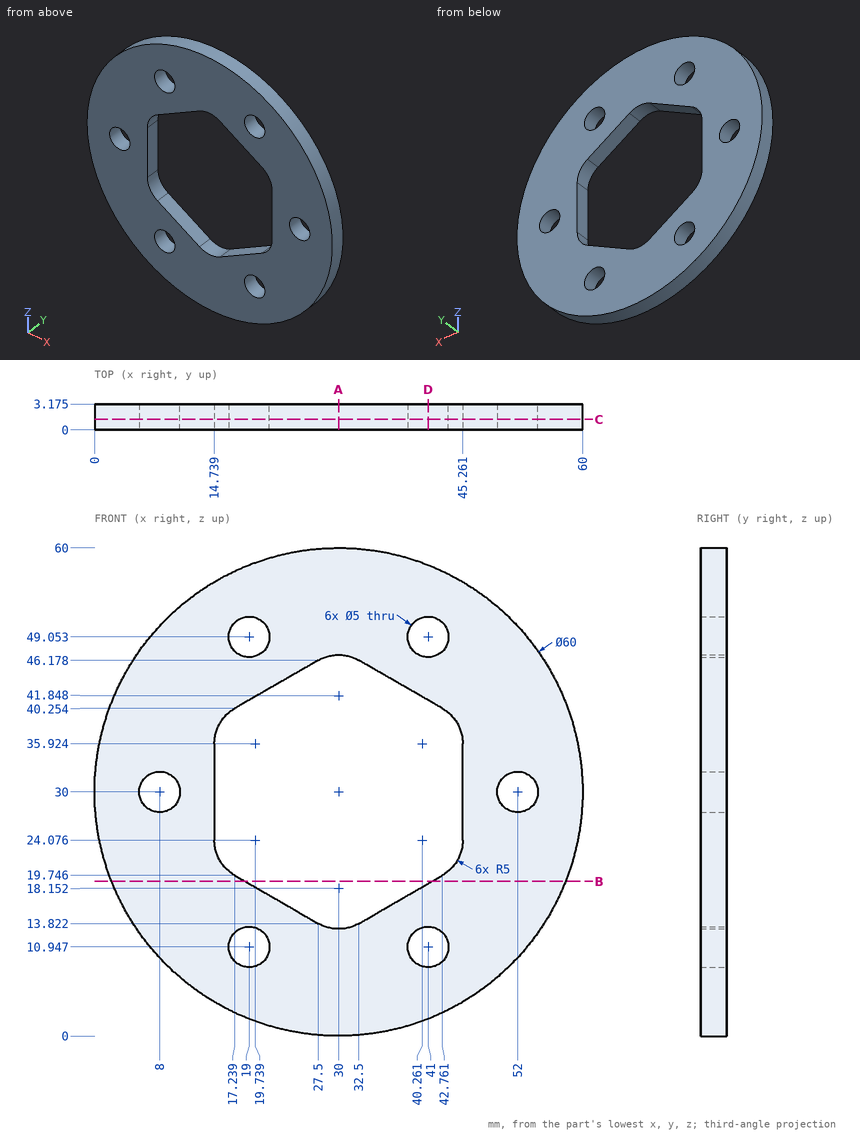
Job drawing, mm, ordinate dimensions from the low corner. One solid piece. Coordinates: 2 decimals unless noted, no trailing zeros. Order: outer loops, then holes, each group sorted by start corner. A loop starts at its lowest first (then second) coordinate and runs counter-clockwise, first axis right, second up. Notation, with made-up numbers: (44.25, 5.5) -> (85.25, 5.5) arc R13 ccw to (85.25, 19.5) -> close; hole circle Ø5 at (63.5, -17). An arc over 180 degrees is marked (long way). Answer in a Markdown table with one row per item. Add a question column.
Q1. Band-saw the part on C-C, the plane y = 1.3. List the corners of the cut face in (x, z) (1 decimal), then the cut area to 3 significant figures.
Q2. Band-saw the part on B-B, the plane z = 19. List the corners of the cut face in (x, y) (1 decimal), then the cut area to 3 significant figures.
Q3. Band-saw the part on A-A, the plane x = 30. List the corners of the cut face in (y, z) (1 decimal).
Q4. Band-saw the part on D-D, the plane x = 41. List the corners of the cut face in (y, z) (1 decimal).
Q5. Drop flat-ended pins along their axis: pin 1 (1 mm diameter, centred on y = 2, z = 31, fed in from -X); pin 2 (1 mm diameter, centred on x = 9.5, y = 3, fed in from +Z); pin 3 (4 mm diameter, centred on x = 19, z = 49.05, fed in from -Y) (3 decimals); pin 4 (1 mm diameter, centred on y = 2, z = 49.5, fed in from -X) (1 decimal). Give the stop position or say it passes through.
Q6. Wall check: line 1 along Z through (x, y) = (19, 0.95); line 2 along X through (y, z) = (1.75, 11) (1 decimal); line 3 along X through (y, z) = (0.9, 28.5). Give the ranges that are in metal, low to high. Write a range as [from, to].
Answers follow:
| question | item | result |
|---|---|---|
| 1 | outline | circle Ø60 at (30, 30); hole circle Ø5 at (8, 30); hole (14.7, 24.1) arc R5 ccw to (17.2, 19.7) -> (27.5, 13.8) arc R5 ccw to (32.5, 13.8) -> (42.8, 19.7) arc R5 ccw to (45.3, 24.1) -> (45.3, 35.9) arc R5 ccw to (42.8, 40.3) -> (32.5, 46.2) arc R5 ccw to (27.5, 46.2) -> (17.2, 40.3) arc R5 ccw to (14.7, 35.9) -> close; hole circle Ø5 at (19, 10.9); hole circle Ø5 at (19, 49.1); hole circle Ø5 at (41, 10.9); hole circle Ø5 at (41, 49.1); hole circle Ø5 at (52, 30) |
| 1 | area | 1,910 mm^2 |
| 2 | outline | (2.1, 0) -> (18.5, 0) -> (18.5, 3.2) -> (2.1, 3.2) -> close; (41.5, 0) -> (57.9, 0) -> (57.9, 3.2) -> (41.5, 3.2) -> close |
| 2 | area | 104 mm^2 |
| 3 | outline | (0, 0) -> (3.2, 0) -> (3.2, 13.2) -> (0, 13.2) -> close; (0, 46.8) -> (3.2, 46.8) -> (3.2, 60) -> (0, 60) -> close |
| 4 | outline | (0, 2.1) -> (3.2, 2.1) -> (3.2, 8.4) -> (0, 8.4) -> close; (0, 13.4) -> (3.2, 13.4) -> (3.2, 18.7) -> (0, 18.7) -> close; (0, 41.3) -> (3.2, 41.3) -> (3.2, 46.6) -> (0, 46.6) -> close; (0, 51.6) -> (3.2, 51.6) -> (3.2, 57.9) -> (0, 57.9) -> close |
| 5 | pin 1 | x = 0 |
| 5 | pin 2 | z = 52.36 |
| 5 | pin 3 | through |
| 5 | pin 4 | x = 6.8 |
| 6 | line 1 | [2.09, 8.45], [13.45, 18.73], [41.27, 46.55], [51.55, 57.91] |
| 6 | line 2 | [6.8, 16.5], [21.5, 38.5], [43.5, 53.2] |
| 6 | line 3 | [0.04, 6], [10, 14.74], [45.26, 50], [54, 59.96] |
